Input: part model. Units: mm. Frame: model coordinates. A direction names the side the tool comes from. Round coordinates to 2 decimals unless told otherwise and drop trailing zeros. Loops run counter-clockwise (first coordinate to the right, second up) from the corner with the lowest first, then second, coordinate; pieces in that order, holes last. Notation, with made-up numbers: (37.25, 14) -> (86.25, 14) arc R13 cw to (86.25, 34) -> close; hole circle Ø7 at (27.5, 19). An arc over 180 degrees is marked (long way). Answer in a Markdown table with one row per item. Add a question column.
Q1. Mould query, pull axis Y, two halves, no side actions, for faces 5 (the face through (-5.02, -26.21, 0.64)), 6 (the face through (-11, 3, 6.35)), 7 (the face through (6.097, -43.258, 3.148)). Classes: pulls with the +Y half, pulls with the -Y half, needs draft (parallel to the pull), parting line crosses it, or undercut.
Q2. Section A-A, the plane y = 0. Output: boundary loops of the cut face in (x, z), and give its area (3 significant figures).
Q3. Section B-B, the plane x = -26.5. Output: boundary loops of the cut face in (y, z), and give its area (3 significant figures).
Q4. Pin query (flat end, axial travel): pin 1 (1.5 mm diameter, centred on y = -15, z = 2.5, fed in from +X); pin 2 (1.5 mm diameter, centred on x = 10, z = 5.5, fed in from -Y); pin 3 (1.9 mm diameter, centred on x = -29.5, z = 3, fed in from -Y). Return the tip coordinate at first contact, or that it passes through.
Q5. Reachability of faces 1 (the face through (-20.097, -18.39, 3.148)), 2 (the face through (33.67, -15.84, 5.71)), 3 (the face through (-5.88, 26.6, 3.15)), 4 (the face through (21.558, 0, 3)) from +Z, -Z, +X, -X, +Y, -Y: full face, straight path, thin tool, end or side. Return the list, or none.
Q6. Ray query, L1, parallel to Y at x = 23, z = 1.75; L2, parallel to X at y = -16.5, z = 4; L3, parallel to Y at x = 6.5, z = 6.25. Return the intervals inside material, ascending. Write a range as from..to.
Q7. Section C-C, the plane z = 3.25. Output: boundary loops of the cut face in (x, y).
Q8. Section D-D, the plane x = -36. Output: boundary loops of the cut face in (y, z), and give its area (3 significant figures).
```python
from build123d import *

# Parameters (mm, degrees)
F1_DEPTH = 6.35
F2_D     = 21.844
F3_SIZE  = 1.27


with BuildPart() as f1:
    # F0 (on Top) → F1 (new body)
    with BuildSketch(Plane.XY):
        Polygon((12.189453, -42.452835), (21.42998, -37.117814), (30.670507, -31.782793), (38.053966, -22.170926), (30.270115, -8.688899), (21.557817, -7.71608), (21.557817, 7.71608), (30.270115, 8.688899), (38.053966, 22.170926), (30.670507, 31.782793), (21.42998, 37.117814), (12.189453, 42.452835), (0.173602, 44.041164), (-7.61025, 30.559138), (-4.096587, 22.527657), (-17.46123, 14.811577), (-22.659865, 21.870239), (-38.227568, 21.870238), (-42.85996, 10.670042), (-42.85996, 0), (-42.85996, -10.670042), (-38.227568, -21.870238), (-22.659865, -21.870239), (-17.46123, -14.811577), (-4.096587, -22.527657), (-7.61025, -30.559138), (0.173602, -44.041164), align=None)
    extrude(amount=F1_DEPTH)

    # F2 (through all)
    with Locations(Plane(origin=(0, 0, 0), x_dir=(1, 0, 0), z_dir=(0, 0, -1))):
        with Locations((13.49248, 23.369661), (0, 0), (-26.98496, 0), (13.49248, -23.369661)):
            Hole(F2_D / 2)

    # F3
    f3_edges = [f1.edges().sort_by_distance(p)[0] for p in [
        (-3.718324, 37.300151, 0),
        (-3.718324, 37.300151, 6.35),
        (6.181528, 43.247, 6.35),
        (6.181528, 43.247, 0),
        (21.42998, 37.117814, 6.35),
        (21.42998, 37.117814, 0),
        (34.362237, 26.97686, 0),
        (34.362237, 26.97686, 6.35),
        (34.16204, 15.429912, 0),
        (34.16204, 15.429912, 6.35),
        (25.913966, 8.20249, 0),
        (25.913966, 8.20249, 6.35),
        (21.557817, 0, 0),
        (21.557817, 0, 6.35),
        (25.913966, -8.20249, 0),
        (25.913966, -8.20249, 6.35),
        (34.16204, -15.429912, 0),
        (34.16204, -15.429912, 6.35),
        (34.362237, -26.97686, 0),
        (34.362237, -26.97686, 6.35),
        (21.42998, -37.117814, 0),
        (21.42998, -37.117814, 6.35),
        (6.181528, -43.247, 0),
        (6.181528, -43.247, 6.35),
        (-3.718324, -37.300151, 0),
        (-3.718324, -37.300151, 6.35),
        (-5.853418, -26.543398, 0),
        (-5.853418, -26.543398, 6.35),
        (-10.778908, -18.669617, 0),
        (-10.778908, -18.669617, 6.35),
        (-20.060547, -18.340908, 6.35),
        (-20.060547, -18.340908, 0),
        (-30.443716, -21.870239, 6.35),
        (-30.443716, -21.870239, 0),
        (-40.543764, -16.27014, 6.35),
        (-40.543764, -16.27014, 0),
        (-42.85996, 0, 6.35),
        (-42.85996, 0, 0),
        (-40.543764, 16.27014, 6.35),
        (-40.543764, 16.27014, 0),
        (-30.443716, 21.870239, 6.35),
        (-30.443716, 21.870239, 0),
        (-20.060547, 18.340908, 6.35),
        (-20.060547, 18.340908, 0),
        (-10.778908, 18.669617, 6.35),
        (-10.778908, 18.669617, 0),
        (-5.853418, 26.543398, 0),
        (-5.853418, 26.543398, 6.35),
    ]]
    chamfer(f3_edges, length=F3_SIZE)


solid = f1.part
```
Answer block:
| question | item | result |
|---|---|---|
| 1 | face 5 | undercut |
| 1 | face 6 | needs draft |
| 1 | face 7 | pulls with the -Y half |
| 2 | outline | (-42.86, 1.27) -> (-41.59, 0) -> (-37.91, 0) -> (-37.91, 6.35) -> (-41.59, 6.35) -> (-42.86, 5.08) -> close; (-16.06, 0) -> (-10.92, 0) -> (-10.92, 6.35) -> (-16.06, 6.35) -> close; (10.92, 0) -> (20.29, 0) -> (21.56, 1.27) -> (21.56, 5.08) -> (20.29, 6.35) -> (10.92, 6.35) -> close |
| 2 | area | 128 mm^2 |
| 3 | outline | (-21.87, 1.27) -> (-20.6, 0) -> (-10.91, 0) -> (-10.91, 6.35) -> (-20.6, 6.35) -> (-21.87, 5.08) -> close; (10.91, 0) -> (20.6, 0) -> (21.87, 1.27) -> (21.87, 5.08) -> (20.6, 6.35) -> (10.91, 6.35) -> close |
| 3 | area | 136 mm^2 |
| 4 | pin 1 | x = 34.35 |
| 4 | pin 2 | y = -42.82 |
| 4 | pin 3 | y = -21.87 |
| 5 | face 1 | +Z, -Z, -Y |
| 5 | face 2 | +Z, +X |
| 5 | face 3 | +Z, -Z, -X |
| 5 | face 4 | +Z, -Z, +X |
| 6 | L1 | -36.21..-28.75, -17.99..-7.88, 7.88..17.99, 28.75..36.21 |
| 6 | L2 | -40.45..-18.7, -14.54..5, 21.98..34.78 |
| 6 | L3 | -42.02..-31.76, -14.98..-8.78, 8.78..14.98, 31.76..42.02 |
| 7 | outline | (-42.86, -10.67) -> (-38.23, -21.87) -> (-22.66, -21.87) -> (-17.46, -14.81) -> (-4.1, -22.53) -> (-7.61, -30.56) -> (0.17, -44.04) -> (12.19, -42.45) -> (30.67, -31.78) -> (38.05, -22.17) -> (30.27, -8.69) -> (21.56, -7.72) -> (21.56, 7.72) -> (30.27, 8.69) -> (38.05, 22.17) -> (30.67, 31.78) -> (12.19, 42.45) -> (0.17, 44.04) -> (-7.61, 30.56) -> (-4.1, 22.53) -> (-17.46, 14.81) -> (-22.66, 21.87) -> (-38.23, 21.87) -> (-42.86, 10.67) -> close; hole circle Ø21.84 at (-26.98, 0); hole circle Ø21.84 at (0, 0); hole circle Ø21.84 at (13.49, -23.37); hole circle Ø21.84 at (13.49, 23.37) |
| 8 | outline | (-21.87, 1.27) -> (-20.6, 0) -> (-6.17, 0) -> (-6.17, 6.35) -> (-20.6, 6.35) -> (-21.87, 5.08) -> close; (6.17, 0) -> (20.6, 0) -> (21.87, 1.27) -> (21.87, 5.08) -> (20.6, 6.35) -> (6.17, 6.35) -> close |
| 8 | area | 196 mm^2 |
